```python
from build123d import *

# Parameters (mm, degrees)
SKETCH2_OUTSIDE_W  = 34.202
SKETCH2_OUTSIDE_H  = 34.202
CUT_EXTRUDE1_DEPTH = 78.047514026
CHAMFER1_SIZE      = 0.508


with BuildPart() as part:
    # Sketch1 → Revolve1 (revolve)
    with BuildSketch(Plane(origin=(0, 0, 0), x_dir=(0, 0, -1), z_dir=(1, 0, 0)), mode=Mode.PRIVATE) as revolve1_sk:
        Polygon((0, 0), (0, 6.35), (1.27, 6.35), (1.27, 5.842), (2.2606, 5.842), (2.2606, 6.875), (22.9108, 6.875), (22.9108, 7.9375), (37.846, 7.9375), (37.846, 6.875), (37.846, 6.35), (49.9491, 6.35), (49.9491, 7.9375), (70.4342, 7.9375), (70.4342, 6.875), (78.486, 6.875), (78.486, 0), align=None)
    revolve(revolve1_sk.sketch.rotate(Axis((0, 0, 0), (0, 0, 1)), 90), axis=Axis((0, 0, 0), (0, 0, 1)))

    # Sketch2 outside → Cut-Extrude1 (cut, through all)
    with BuildSketch(Plane.XY.offset(-2.2606)):
        Rectangle(SKETCH2_OUTSIDE_W, SKETCH2_OUTSIDE_H)
        Polygon((3.666174209, 6.35), (-3.666174209, 6.35), (-7.332348419, 0), (-3.666174209, -6.35), (3.666174209, -6.35), (7.332348419, 0), align=None, mode=Mode.SUBTRACT)
    extrude(amount=-CUT_EXTRUDE1_DEPTH, mode=Mode.SUBTRACT)

    # Chamfer1
    chamfer1_edges = [part.edges().sort_by_distance(p)[0] for p in [
        (6.35, 0, 0),
    ]]
    chamfer(chamfer1_edges, length=CHAMFER1_SIZE)


solid = part.part
```
Part model, mm, in its own coordinate system. A direction names the side the tool comes from. Give positions to 0.01 mm unless a question says otherwise; leave off trailing zeros. Order: outer loops, then holes, each group sorted by start corner. A loop starts at its lowest first (then second) coordinate and runs counter-clockwise, first axis right, second up. Notation, with made-up numbers: (57.5, 79) - (63.5, 79) arc R9 cw to (63.5, 88) - close; hole circle Ø5 at (56, 73.25). An arc over 180 degrees is marked (long way). Use one line per item in the form item = value.
Item 1: Slice it at C-C on z = -45. Give the cut face in (x, y), and give its area (3 significant figures).
Solution:
outline = circle Ø12.7 at (0, 0)
area = 127 mm2
Item 2: Two-plate mould, pull along Z, no slides. Class faces 6 (the face through (-2, -6, -2.261)), 7 (the face through (-5.525, -3.131, -19.804)), 8 (the face through (-3, -6, -49.949)), 9 (the face through (0, 0, 0)): released by +Z, released by -Z, zero draft, split by the parting line, or undercut.
Solution:
face_6 = undercut
face_7 = zero draft
face_8 = undercut
face_9 = released by +Z
Item 3: Probe probe 1 along X at (y, z) = (3.25, -31.5); probe 2 along Y at (x, z) = (-5.5, -32); probe 3 along X at (y, z) = (-0.75, -15.5). List the from-to ranges inside material, lowest first. Write a range as from..to.
Solution:
probe_1 = -5.46..5.46
probe_2 = -3.17..3.17
probe_3 = -6.83..6.83
Item 4: Which spindle directions (+Z, -Z, +X, -X, +Y, -Y) get a long thin tool onto all of the face, cutting with end or side? Do faces 1 (the face through (6.875, -0.013, -12.73)), 2 (the face through (3.448, 5.948, -74.516)), 3 (the face through (-6.875, 0.013, -12.73)), 4 (the face through (3, 6, -49.949)), 5 (the face through (3, -6, -49.949)). Say none if no direction does.
Solution:
face_1 = +Z, +X
face_2 = -Z, +X, +Y
face_3 = +Z, -X
face_4 = +X, +Y
face_5 = +X, -Y
Item 5: Pin check, flat tips, straight feed: pin 1 Ø5 at (y, z) = (-1, -53) entering from -X; pin 2 Ø5 at (y, z) = (5, -55.5) entering from +X; pin 3 Ø1.5 at (x, z) = (-4, -12.5) entering from -Y. Stop position of each tip, or through.
Solution:
pin_1 = -7.33
pin_2 = 5.89
pin_3 = -6.06
Item 6: Slice it at A-A on z = -19. Give the cut face in (x, y) (3 decimals), and give its area (3 significant figures).
Solution:
outline = (-6.817, -0.893) - (-4.182, -5.457) arc R6.875 ccw to (-2.635, -6.35) - (2.635, -6.35) arc R6.875 ccw to (4.182, -5.457) - (6.817, -0.893) arc R6.875 ccw to (6.817, 0.893) - (4.182, 5.457) arc R6.875 ccw to (2.635, 6.35) - (-2.635, 6.35) arc R6.875 ccw to (-4.182, 5.457) - (-6.817, 0.893) arc R6.875 ccw to start
area = 137 mm2
Item 7: Slice it at B-B on z = -32. Give the cut face in (x, y).
Solution:
outline = (-7.33, 0) - (-3.67, -6.35) - (3.67, -6.35) - (7.33, 0) - (3.67, 6.35) - (-3.67, 6.35) - close
